Source: three-view drawing plus pictorial views. Frame: mm from the lowest corner of the part. A direction names the side the tool comes from. Coordinates: 2 decimals unless noted, no trailing zeros. Write each loop counter-clockwise with the first axis right and the second up, starting at its lowest first coordinate (ties: lowest second). Pieces come first, ordered by that corner, then holes. Notation, with made-up numbers: (10, 0.5) - (69, 0.5) arc R23 ccw to (69, 28.5) - close; hole circle Ø5 at (-21.75, 46). An arc over 180 degrees is marked (long way). Put each result on its own line as item: value.
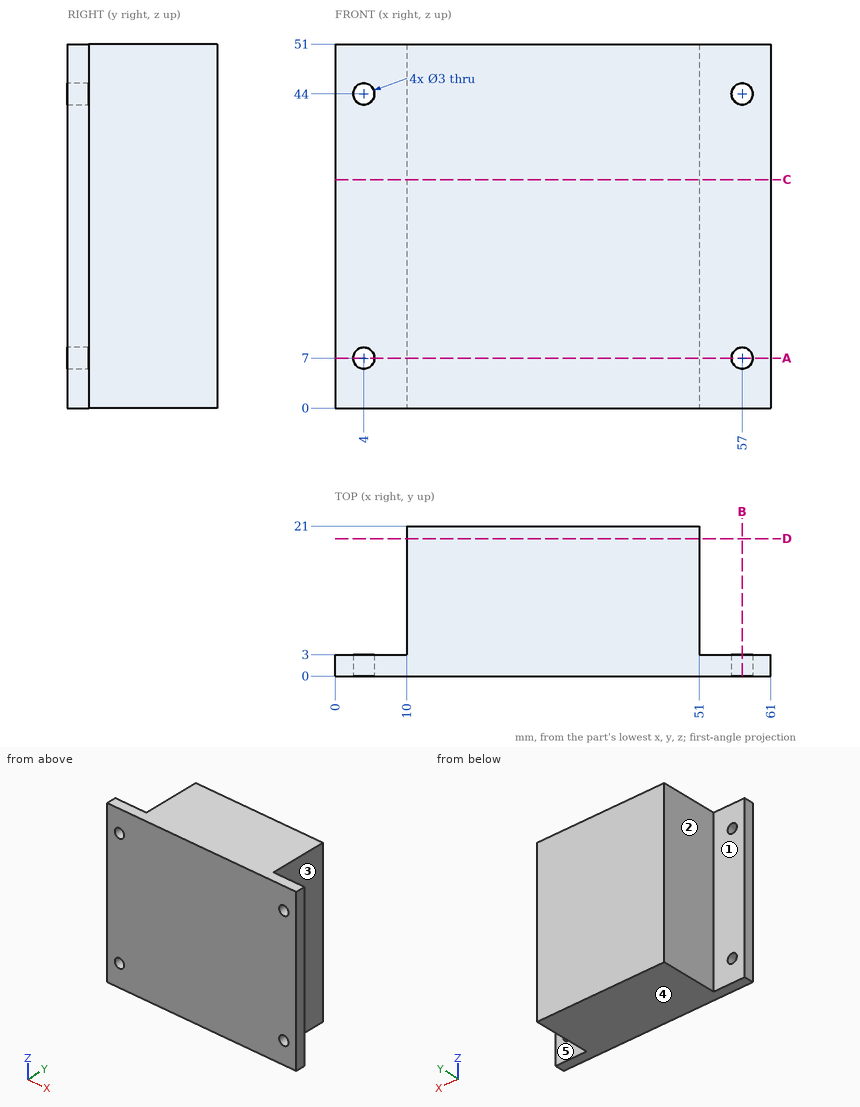
1. Section query A-A (z = 7). Return loops of the section in (x, y), then the cut area to 3 significant figures.
Answer below:
outline: (0, 0) - (2.5, 0) - (2.5, 3) - (0, 3) - close; (5.5, 0) - (55.5, 0) - (55.5, 3) - (51, 3) - (51, 21) - (10, 21) - (10, 3) - (5.5, 3) - close; (58.5, 0) - (61, 0) - (61, 3) - (58.5, 3) - close
area: 903 mm²
2. Pin query (flat end, axial travel): pin 1 Ø5 at (y, z) = (7, 19) entering from +X; pin 2 Ø2.5 at (x, z) = (4, 7) entering from +Y; pin 3 Ø5 at (x, z) = (7, 28) entering from +Y; pin 4 Ø5.5 at (y, z) = (10.5, 27) entering from -X. Return the tip coordinate at first contact, or that it passes through.
Answer below:
pin 1: stops at x = 51
pin 2: passes through
pin 3: stops at y = 3
pin 4: stops at x = 10
3. Ray query, probe 1 along Z at (x, y) = (4, 1.65); probe 2 along X at (y, z) = (0.8, 7); probe 3 along X at (y, z) = (7, 9). Return the intervals inside material, ascending. Write a range as from..to.
Answer below:
probe 1: z = 0..5.5, 8.5..42.5, 45.5..51
probe 2: x = 0..2.5, 5.5..55.5, 58.5..61
probe 3: x = 10..51
4. Section query C-C (z = 32). Return loops of the section in (x, y), then the cut area to 3 significant figures.
Answer below:
outline: (0, 0) - (61, 0) - (61, 3) - (51, 3) - (51, 21) - (10, 21) - (10, 3) - (0, 3) - close
area: 921 mm²
5. Section query B-B (x = 57). Return loops of the section in (y, z).
Answer below:
outline: (0, 0) - (3, 0) - (3, 5.5) - (0, 5.5) - close; (0, 8.5) - (3, 8.5) - (3, 42.5) - (0, 42.5) - close; (0, 45.5) - (3, 45.5) - (3, 51) - (0, 51) - close
6. Set-up query: the marked faces 4 and 5. Return all of +Z, -Z, +X, -X, +Y, -Y with unobstructed straight access to the full face (end or side cutting, diameter ignored); none if empty.
Answer below:
face 4: -Z, +X, -X, +Y, -Y
face 5: +Z, -Z, +X, +Y
7. Mould query, pull axis X, two halves, no side actions, for the marked faces 1, 2 and 3. Classes: +X half, -X half, draft (parallel to the pull), parting line (faces both ways), or undercut.
Answer below:
face 1: draft
face 2: -X half
face 3: +X half
8. Section query D-D (y = 19.25). Return loops of the section in (x, z).
Answer below:
outline: (10, 0) - (51, 0) - (51, 51) - (10, 51) - close
